The model under review builds one solid part; all positions refer to its coordinate system, in mm. A direction names the side the tool comes from. Round coordinates to 2 decimals unless told otherwise and drop trailing zeros. Write each loop counter-clockwise with the first axis right and the second up, starting at its lowest first coordinate (ties: lowest second). Pieces come first, ordered by that corner, then holes.
Item 1: Clearance check with a flat-ended pin moving along its axis: pin 1 Ø1 at (y, z) = (-1.5, -1) entering from +X. State where the tip first meets the part, or that it passes through.
Item 2: Add section D-D (x = -0.9). Give the boundary of the cut face in (y, z).
Item 3: Add section C-C (y = 0.5). Give the boundary of the cut face in (x, z).
Item 4: Draft analysis for pull direction Z (two halves, no side actions). For faces 4 (the face through (0.735, 2.465, -1.25)), 5 (the face through (-1.45, 2, 0)), 6 (the face through (-1, 3, 0)), state which applies: +Z half, -Z half, draft (parallel to the pull), parting line (faces both ways), or undercut.
Item 5: Add section A-A (y = 2.5). Give the boundary of the cut face in (x, z).
Item 6: Add section B-B (z = 0). Give the boundary of the cut face in (x, y).
Item 7: To check wall thickness, follow L1, parallel to X at y = 4.1, z = 0; L2, parallel to Y at x = -0.1, z = 0.4; L3, parallel to Y at x = -1.1, z = 0.3. State the ranges of each line that lie inside material, in increasing order.
Item 8: Machinability: for faces 1 (the face through (0, 2, 0)), 2 (the face through (-1, -2, 0)), 3 (the face through (0, -4, 0)), which of the approach directions +Z, -Z, +X, -X, +Y, -Y give a long, thin tool a straight path to every point of the face, cutting with its end or side? Answer none if there is none.
```python
from build123d import *

# Parameters (mm, degrees)
SKETCH_1_R           = 1
EXTRUDE_1_DEPTH      = 5
EXTRUDE_2_DEPTH      = 4
EXTRUDE_2_DEPTH_BACK = 2
SKETCH_2_R           = 1


with BuildPart() as part:
    # 草图1 → 凸台-拉伸1 (new body)
    with BuildSketch(Plane(origin=(0, 0, 0), x_dir=(1, 0, 0), z_dir=(0, 1, 0))):
        Polygon((0, 1.674315781), (-1.45, 0.83715789), (-1.45, -0.83715789), (0, -1.674315781), (1.45, -0.83715789), (1.45, 0.83715789), align=None)
        with Locations(Location((0, 0, 0), (0, 0, 270))):
            Circle(SKETCH_1_R, mode=Mode.SUBTRACT)
    extrude(amount=EXTRUDE_1_DEPTH)

    # 草图2 → 凸台-拉伸2 (add, two sides: drawn at the far end of the back side and taken through both)
    with BuildSketch(Plane.XZ.offset(-EXTRUDE_2_DEPTH_BACK)):
        with Locations(Location((0, 0, 0), (0, 0, 270))):
            Circle(SKETCH_2_R)
    extrude(amount=EXTRUDE_2_DEPTH + EXTRUDE_2_DEPTH_BACK)


solid = part.part
```
Numbers:
1. pin 1: stops at x = 0.87
2. outline: (-4, -0.44) - (0, -0.44) - (0, -1.15) - (5, -1.15) - (5, -0.44) - (2, -0.44) - (2, 0.44) - (5, 0.44) - (5, 1.15) - (0, 1.15) - (0, 0.44) - (-4, 0.44) - close
3. outline: (-1.45, -0.84) - (0, -1.67) - (1.45, -0.84) - (1.45, 0.84) - (0, 1.67) - (-1.45, 0.84) - close
4. face 4: -Z half
4. face 5: draft
4. face 6: undercut
5. outline: (-1.45, -0.84) - (0, -1.67) - (1.45, -0.84) - (1.45, 0.84) - (0, 1.67) - (-1.45, 0.84) - close; hole circle Ø2 at (0, 0)
6. outline: (-1.45, 0) - (-1, 0) - (-1, -4) - (1, -4) - (1, 0) - (1.45, 0) - (1.45, 5) - (1, 5) - (1, 2) - (-1, 2) - (-1, 5) - (-1.45, 5) - close
7. L1: x = -1.45 to -1, 1 to 1.45
7. L2: y = -4 to 2
7. L3: y = 0 to 5
8. face 1: +Y
8. face 2: -Y
8. face 3: +Z, -Z, +X, -X, -Y
